CAD build for the part. Positions are in the model's coordinates, mm. A direction names the side the tool comes from. Give positions to 0.01 mm unless a question says otherwise; leave off trailing zeros. Loops run counter-clockwise (first coordinate to the right, second up) from the corner with the lowest first, then second, coordinate; pieces in that order, holes last. Notation, with made-up numbers: (-20, -11) -> (-16, -11) arc R13 cw to (-16, 10) -> close; hole circle Ø3 at (-7, -37.75). An arc over 180 degrees is marked (long way). Write each question's results on one line, items separated by ' | '. Start each with the question number.
```python
from build123d import *

# Parameters (mm, degrees)
F1_W     = 279.4
F1_H     = 228.6
F1_W_2   = 304.8
F1_H_2   = 254
F2_DEPTH = 9.525
F3_W     = 279.4
F3_H     = 228.6
F4_DEPTH = 9.525
F5_R     = 6.35
F6_DEPTH = 33.178601


with BuildPart() as f2:
    # F1 (on face) → F2 (new body)
    with BuildSketch(Plane.XY):
        Rectangle(F1_W, F1_H)
        Rectangle(F1_W_2, F1_H_2)
        Rectangle(F1_W, F1_H, mode=Mode.SUBTRACT)
    extrude(amount=F2_DEPTH)

    # F3 (on face) → F4 (join, symmetric)
    with BuildSketch(Plane.XY.offset(9.525)):
        Rectangle(F3_W, F3_H)
    extrude(amount=F4_DEPTH, both=True)

    # F5 (on face) → F6 (cut, symmetric)
    with BuildSketch(Plane.XY.offset(19.05)):
        Circle(F5_R)
    extrude(amount=F6_DEPTH, both=True, mode=Mode.SUBTRACT)


solid = f2.part
```
Q1. Saw through at B-B, the plane x = 0. List the corners of the cut face in (y, z) (3 decimals).
Q2. Mould opens along X. For faces 4 (the face through (-2, 27, 19.05)), 5 (the face through (139.7, -2, 14)), 6 (the face through (-139.7, -2, 14)), 7 (the face through (-1.38, -6.2, 9.66)) say: pulls with the +X half, pulls with the -X half, needs draft (parallel to the pull), parting line crosses it, or undercut.
Q3. Which spindle directions (+Z, -Z, +X, -X, +Y, -Y) get a long thin tool onto all of the face, cutting with end or side? Do faces 1 (the face through (-2, 114.3, 14)), 2 (the face through (-2, -114.3, 14)), 3 (the face through (-2, 127, 5)). Say none if no direction does.
Q4. Saw through at C-C, the plane z = 13.75. List the corners of the cut face in (x, y), then the cut area to 3 significant figures.
Q5. Wall check: L1, parallel to Y at x = 0, z = 11; L2, parallel to Y at x = 0, z = 4.75; L3, parallel to X at y = -25, z = 12.25. Give the ranges that are in metal, low to high.
Q6. Drop flat-ended pins along their axis: pin 1 (3 mm diameter, centred on x = 0, z = 14.5, fed in from +Y); pin 2 (1.5 mm diameter, centred on x = -92.5, z = 14.5, fed in from -Y); pin 3 (1.5 mm diameter, centred on x = 4.5, y = -74, fed in from -Z); pin 4 (1 mm diameter, centred on y = 87.5, z = 11, fed in from +X). Give the stop position or say it passes through.
Q7. Saw through at A-A, the plane y = 0. List the corners of the cut face in (x, z) (3 decimals).
Q8. Saw through at D-D, the plane x = 92.5. List the corners of the cut face in (y, z) (3 decimals).
Answer block:
1) outline: (-127, 0) -> (-6.35, 0) -> (-6.35, 19.05) -> (-114.3, 19.05) -> (-114.3, 9.525) -> (-127, 9.525) -> close; (6.35, 0) -> (127, 0) -> (127, 9.525) -> (114.3, 9.525) -> (114.3, 19.05) -> (6.35, 19.05) -> close
2) face 4: needs draft | face 5: pulls with the +X half | face 6: pulls with the -X half | face 7: undercut
3) face 1: +Z, +X, -X, +Y | face 2: +Z, +X, -X, -Y | face 3: +Z, -Z, +X, -X, +Y
4) outline: (-139.7, -114.3) -> (139.7, -114.3) -> (139.7, 114.3) -> (-139.7, 114.3) -> close; hole circle Ø12.7 at (0, 0) | area: 63,700 mm2
5) L1: y = -114.3 to -6.35, 6.35 to 114.3 | L2: y = -127 to -6.35, 6.35 to 127 | L3: x = -139.7 to 139.7
6) pin 1: stops at y = 114.3 | pin 2: stops at y = -114.3 | pin 3: stops at z = 0 | pin 4: stops at x = 139.7
7) outline: (-152.4, 0) -> (-6.35, 0) -> (-6.35, 19.05) -> (-139.7, 19.05) -> (-139.7, 9.525) -> (-152.4, 9.525) -> close; (6.35, 0) -> (152.4, 0) -> (152.4, 9.525) -> (139.7, 9.525) -> (139.7, 19.05) -> (6.35, 19.05) -> close
8) outline: (-127, 0) -> (127, 0) -> (127, 9.525) -> (114.3, 9.525) -> (114.3, 19.05) -> (-114.3, 19.05) -> (-114.3, 9.525) -> (-127, 9.525) -> close
